Autodesk Inventor part; units mm, degrees
ref_plane "YZ Plane" through (0, 0, 0) normal (1, 0, 0) x (0, 1, 0)
ref_plane "XZ Plane" through (0, 0, 0) normal (0, 1, 0) x (-1, 0, 0)
ref_plane "XY Plane" through (0, 0, 0) normal (0, 0, 1) x (1, 0, 0)
sketch "Эскиз1" plane through (0, 0, 0) normal (0, 1, 0) x (-1, 0, 0)
  circle A0 centre (0, 0) radius 8.75
  circle A1 centre (0, 0) radius 2.6
  circle A2 centre (0, 0) radius 4
  circle A3 centre (0, 0) radius 7.25
  point P0 (-0.75, 3.9291)
  point P1 (-0.6797, 7.2181)
  point P2 (0.6797, 7.2181)
  point P3 (0.75, 3.9291)
  dimension "d1" = 5.2
  dimension "d2" = 8
  dimension "d41" = 17.5
  dimension "d43" = 1.5
extrude "Выдавливание1" add sketch "Эскиз1" along normal blind 8 contours A0
extrude "Выдавливание7" add sketch "Эскиз1" along normal blind 6 contours A2
extrude "Выдавливание8" add sketch "Эскиз1" along normal blind 1.75 contours A3
properties part number "Колесо"
Can you work these out from the model? Positions are in its coordinate system, mm. A direction names the side the tool comes from. Coordinates: 2 decimals unless noted, no trailing zeros. Loops run counter-clockwise (first coordinate to the right, second up) from the corner with the lowest first, then second, coordinate; pieces in that order, holes last. Notation, with made-up numbers: (35, -3.75) - (80, -3.75) arc R29 cw to (80, 24.25) - close; hole circle Ø8 at (1.5, -10.75). An arc over 180 degrees is marked (long way). Answer as a JSON object with one key per item and string values. Group by question number.
Item 1: If we mould it in two halves opening along X, with no side actions, what happens to faces 1 (the face through (6.944, 3.944, 5.324)), 2 (the face through (3, 8, 7)), 3 (the face through (0.867, 3.845, 3.905))? For each: released by +X, released by -X, zero draft, split by the parting line, or undercut.
Item 2: If I drill on L1, parallel to Z at x = 0, y = 4.65; L2, parallel to Z at x = 0, y = 6.5; L3, parallel to X at y = 2.5, z = 3.25, over which ranges is the centre line in solid material (lowest first)? Write a range as from..to.
Item 3: If we section it at D-D (x = 3.5): List the corners of the cut face in (y, z) for me.
Item 4: If we section it at C-C (y = 3): List the corners of the cut face in (x, z) for me.
Item 5: If we section it at B-B (x = 0): List the corners of the cut face in (y, z) for me.
Item 6: For pin 1 (3 mm diameter, centred on x = 4.5, y = 1, fed in from -Z); pin 2 (2 mm diameter, centred on x = -3.5, z = -3.5, fed in from +Y); pin 3 (1.5 mm diameter, centred on y = 4.5, z = 3, fed in from -X), each with a flat end and sliding along its axis, tell me the tip position at first contact or that it passes through.
Item 7: If we section it at A-A (z = 0): List the corners of the cut face in (x, y) for me, plus the area to 3 significant figures.
Item 8: On a 3-axis mill with a long thin cutter (end or side, diameter ignored), from which of +Z, -Z, +X, -X, +Y, -Y can I reach the whole of each face in a straight line? I mean faces 4 (the face through (0.338, 2.958, -2.578)), 5 (the face through (-3.35, 4.83, 6.43)). Say none if no direction works.
Returned:
{
 "1": {"face 1": "split by the parting line", "face 2": "zero draft", "face 3": "undercut"},
 "2": {"L1": "z = -8.75..-7.25, -4..-2.6, 2.6..4, 7.25..8.75", "L2": "z = -8.75..-7.25, 7.25..8.75", "L3": "x = -8.12..-6.48, -2.33..2.33, 6.48..8.12"},
 "3": {"outline": "(0, -8.02) - (8, -8.02) - (8, -6.35) - (1.75, -6.35) - (1.75, -1.94) - (6, -1.94) - (6, 1.94) - (1.75, 1.94) - (1.75, 6.35) - (8, 6.35) - (8, 8.02) - (0, 8.02) - close"},
 "4": {"outline": "circle Ø17.5 at (0, 0); circle Ø8 at (0, 0); hole circle Ø14.5 at (0, 0); hole circle Ø5.2 at (0, 0)"},
 "5": {"outline": "(0, -8.75) - (8, -8.75) - (8, -7.25) - (1.75, -7.25) - (1.75, -4) - (6, -4) - (6, -2.6) - (0, -2.6) - close; (0, 2.6) - (6, 2.6) - (6, 4) - (1.75, 4) - (1.75, 7.25) - (8, 7.25) - (8, 8.75) - (0, 8.75) - close"},
 "6": {"pin 1": "stops at z = -8.22", "pin 2": "stops at y = 6", "pin 3": "stops at x = -8.46"},
 "7": {"outline": "(-8.75, 0) - (-2.6, 0) - (-2.6, 6) - (-4, 6) - (-4, 1.75) - (-7.25, 1.75) - (-7.25, 8) - (-8.75, 8) - close; (2.6, 0) - (8.75, 0) - (8.75, 8) - (7.25, 8) - (7.25, 1.75) - (4, 1.75) - (4, 6) - (2.6, 6) - close", "area": "52.2 mm²"},
 "8": {"face 4": "+Y, -Y", "face 5": "+Y"}
}
